Build history of the part. All positions in model axes, mm. Give positions to 0.01 mm unless a question says otherwise; leave off trailing zeros. Loops run counter-clockwise (first coordinate to the right, second up) from the corner with the lowest first, then second, coordinate; pieces in that order, holes last. Notation, with made-up numbers: (78.5, 26.25) -> (131.5, 26.25) arc R31 ccw to (131.5, 56.25) -> close; hole circle Ø7 at (-19, 1). An arc over 180 degrees is marked (long way). Answer as a JSON object with one key per item and string values. Group by question number.
Q1. Band-saw the part on A-A, the plane x = -18.5. Write the cut outline in (y, z).
Q2. Wall check: probe 1 along Z at (x, y) = (-21, 2.15); probe 2 along Z at (x, y) = (-20.25, 2.5); probe 3 along X at (y, z) = (2.45, -16). Give the ranges that are in metal, low to high. Write a range as from..to.
Q3. Band-saw the part on B-B, the plane z = -17.5. Write the cut outline in (x, y), plus the area to 3 significant figures.
Q4. Band-saw the part on C-C, the plane y = 3.7. Write the cut outline in (x, z) (1 decimal), plus the area to 3 significant figures.
Q5. Two-plate mould, pull along X, no slides. Class faces 1 (the flat face through (-21, 1.007, 10)), 2 (the cylindrical face through (-22.05, 2.62, 40.93)), 3 (the cylindrical face through (-27.94, 2.57, -25.12)), 4 (the cylindrical face through (-14.098, 2.572, -24.983)): pulls with the +X half, pulls with the -X half, needs draft (parallel to the pull), parting line crosses it, or undercut.
Q6. Band-saw the part on D-D, the plane x = -15.25. Write the cut outline in (y, z), plus the area to 3 significant figures.
from build123d import *

# Parameters (mm, degrees)
STEM_START                = 1.006990195
STEM_OTHER_SIDE_OUTLINE_R = 3.81
STEM_OTHER_SIDE_DEPTH     = 3.175
SKETCH1_R                 = 1.5875
CUT_EXTRUDE1_DEPTH        = 3.175


# Read off the part's stored shape, not the designer's step: Stem Other Side
with BuildPart() as part:
    # Stem Other Side outline → Stem Other Side (new body)
    with BuildSketch(Plane(origin=(0, 0, 0), x_dir=(1, 0, 0), z_dir=(0, 1, 0)).offset(STEM_START)):
        with BuildLine():
            Line((-20.453203013, 27.656176961), (-21.723203013, 27.656176961))
            ThreePointArc((-21.723203013, 27.656176961), (-28.009382298, 25.052356246), (-30.613203013, 18.766176961))
            Line((-30.613203013, 18.766176961), (-30.613203013, -48.543823039))
            Line((-30.613203013, -48.543823039), (-11.563203013, -48.543823039))
            Line((-11.563203013, -48.543823039), (-11.563203013, 18.766176961))
            ThreePointArc((-11.563203013, 18.766176961), (-14.167023728, 25.052356246), (-20.453203013, 27.656176961))
        make_face()
        with Locations((-21.088203013, 14.956176961)):
            Circle(STEM_OTHER_SIDE_OUTLINE_R, mode=Mode.SUBTRACT)
    extrude(amount=STEM_OTHER_SIDE_DEPTH)

    # Sketch1 → Cut-Extrude1 (cut)
    with BuildSketch(Plane(origin=(0, 4.181990195, 0), x_dir=(1, 0, 0), z_dir=(0, 1, 0))):
        with Locations(Location((-21.088203013, -42.193823039, 0), (0, 0, 270))):
            Circle(SKETCH1_R)
    extrude(amount=-CUT_EXTRUDE1_DEPTH, mode=Mode.SUBTRACT)


solid = part.part
Worked answers:
{
 "1": {"outline": "(1.01, -27.44) -> (4.18, -27.44) -> (4.18, -17.75) -> (1.01, -17.75) -> close; (1.01, -12.16) -> (4.18, -12.16) -> (4.18, 48.54) -> (1.01, 48.54) -> close"},
 "2": {"probe 1": "-27.66..-18.77, -11.15..40.61, 43.78..48.54", "probe 2": "-27.65..-18.67, -11.24..40.85, 43.54..48.54", "probe 3": "-30.61..-24.75, -17.42..-11.56"},
 "3": {"outline": "(-30.61, 1.01) -> (-23.92, 1.01) -> (-23.92, 4.18) -> (-30.61, 4.18) -> close; (-18.25, 1.01) -> (-11.56, 1.01) -> (-11.56, 4.18) -> (-18.25, 4.18) -> close", "area": "42.5 mm2"},
 "4": {"outline": "(-30.6, -18.8) arc R8.9 ccw to (-21.7, -27.7) -> (-20.5, -27.7) arc R8.9 ccw to (-11.6, -18.8) -> (-11.6, 48.5) -> (-30.6, 48.5) -> close; hole circle Ø7.6 at (-21.1, -15); hole circle Ø3.2 at (-21.1, 42.2)", "area": "1,360 mm2"},
 "5": {"face 1": "needs draft", "face 2": "undercut", "face 3": "pulls with the -X half", "face 4": "pulls with the +X half"},
 "6": {"outline": "(1.01, -25.97) -> (4.18, -25.97) -> (4.18, 48.54) -> (1.01, 48.54) -> close", "area": "237 mm2"}
}
